Geometry check sheet. Reference: the model listing, model coordinates, mm. Give positions to 0.01 mm unless a question says otherwise; leave off trailing zeros. Order: outer loops, then holes, each group sorted by start corner. A loop starts at its lowest first (then second) coordinate and runs counter-clockwise, first axis right, second up.
Autodesk Inventor part; units mm, degrees
ref_plane "YZ Plane" through (0, 0, 0) normal (1, 0, 0) x (0, 1, 0)
ref_plane "XZ Plane" through (0, 0, 0) normal (0, 1, 0) x (-1, 0, 0)
ref_plane "XY Plane" through (0, 0, 0) normal (0, 0, 1) x (1, 0, 0)
sketch "Sketch1" plane through (0, 0, 0) normal (0, 0, 1) x (1, 0, 0)
  line L0 (0, 0) -> (0, 6.35)
  line L1 (0, 6.35) -> (97.04, 6.35)
  line L2 (97.04, 6.35) -> (97.04, 0)
  line L3 (97.04, 0) -> (0, 0)
  dimension "d0" = 6.35
  dimension "d1" = 97.04
extrude "Extrusion1" add sketch "Sketch1" along normal blind 332
sketch "Sketch2" plane through (0, 0, 332) normal (0, 0, 1) x (1, 0, 0)
  line L0 (0, 0) -> (16.1733, 0) construction
  line L1 (16.1733, 0) -> (48.52, 0) construction
  line L2 (48.52, 0) -> (80.8667, 0) construction
  line L3 (0, 0) -> (97.04, 0)
  arc A0 (19.3483, 0) -> (12.9983, 0) centre (16.1733, 0) ccw
  arc A1 (51.695, 0) -> (45.345, 0) centre (48.52, 0) ccw
  arc A2 (84.0417, 0) -> (77.6917, 0) centre (80.8667, 0) ccw
  line L4 (12.9983, 0) -> (19.3483, 0)
  line L5 (45.345, 0) -> (51.695, 0)
  line L6 (77.6917, 0) -> (84.0417, 0)
  dimension "d4" = 16.1733
  dimension "d5" = 32.3467
  dimension "d6" = 32.3467
  dimension "d12" = 3.175
  dimension "d13" = 3.175
  dimension "d14" = 3.175
extrude "Extrusion3" cut sketch "Sketch2" against normal through all
sketch "Sketch3" plane through (0, 0, 332) normal (0, 0, 1) x (1, 0, 0)
  arc A0 (19.3483, 0) -> (12.9983, 0) centre (16.1733, 0) ccw
  line L0 (0, 0) -> (0, 6.35) construction
  line L1 (0, 0) -> (0, 3.175) construction
  arc A1 (19.3483, 0) -> (12.9983, 0) centre (16.1733, 0) ccw construction
  line L2 (16.1733, 3.175) -> (12.9983, 3.175)
  line L3 (0, 3.175) -> (6.4992, 3.175) construction
  line L4 (45.345, 0) -> (19.3483, 0) construction
  line L5 (19.3483, 0) -> (32.3467, 0) construction
  circle A2 centre (32.3467, 3.175) radius 1.5
  circle A3 centre (6.4992, 3.175) radius 1.5
  line L6 (51.695, 0) -> (64.6933, 0) construction
  line L7 (77.6917, 0) -> (51.695, 0) construction
  circle A4 centre (64.6933, 3.175) radius 1.5
  line L8 (84.0417, 0) -> (90.5408, 0) construction
  line L9 (97.04, 0) -> (84.0417, 0) construction
  circle A5 centre (90.5408, 3.175) radius 1.5
  dimension "d17" = 3
  dimension "d18" = 3
  dimension "d19" = 3
  dimension "d20" = 3
extrude "Extrusion4" cut sketch "Sketch3" against normal blind 20
sketch "Sketch4" plane through (0, 0, 0) normal (0, 0, -1) x (-1, 0, 0)
  circle A0 centre (-6.4992, 3.175) radius 1.5
  circle A1 centre (-32.3467, 3.175) radius 1.5
  circle A2 centre (-64.6933, 3.175) radius 1.5
  circle A3 centre (-90.5408, 3.175) radius 1.5
  dimension "d23" = 3
  dimension "d24" = 3
  dimension "d25" = 3
  dimension "d26" = 3
extrude "Extrusion5" cut sketch "Sketch4" against normal blind 20
sketch "Sketch5" plane through (0, 0, 332) normal (0, 0, 1) x (1, 0, 0)
  circle A0 centre (64.6933, 3.175) radius 1.5
  circle A1 centre (32.3467, 3.175) radius 1.5
  circle A2 centre (6.4992, 3.175) radius 1.5
  circle A3 centre (90.5408, 3.175) radius 1.5
  arc A4 (51.695, 0) -> (45.345, 0) centre (48.52, 0) ccw
  line L0 (51.695, 0) -> (77.6917, 0)
  arc A5 (84.0417, 0) -> (77.6917, 0) centre (80.8667, 0) ccw
  line L1 (84.0417, 0) -> (97.04, 0)
  line L2 (97.04, 0) -> (97.04, 6.35)
  line L3 (97.04, 6.35) -> (0, 6.35)
  line L4 (0, 6.35) -> (0, 0)
  line L5 (0, 0) -> (12.9983, 0)
  arc A6 (19.3483, 0) -> (12.9983, 0) centre (16.1733, 0) ccw
  line L6 (19.3483, 0) -> (45.345, 0)
extrude "Extrusion6" add sketch "Sketch5" along normal blind 30.87
sketch "Sketch6" plane through (0, 0, 362.87) normal (0, 0, 1) x (1, 0, 0)
  circle A0 centre (90.5408, 3.175) radius 1.5
  circle A1 centre (6.4992, 3.175) radius 1.5
  circle A2 centre (32.3467, 3.175) radius 1.5
  circle A3 centre (64.6933, 3.175) radius 1.5
  arc A4 (51.695, 0) -> (45.345, 0) centre (48.52, 0) ccw
  line L0 (51.695, 0) -> (77.6917, 0)
  arc A5 (84.0417, 0) -> (77.6917, 0) centre (80.8667, 0) ccw
  line L1 (84.0417, 0) -> (97.04, 0)
  line L2 (97.04, 0) -> (97.04, 6.35)
  line L3 (97.04, 6.35) -> (0, 6.35)
  line L4 (0, 6.35) -> (0, 0)
  line L5 (0, 0) -> (12.9983, 0)
  arc A6 (19.3483, 0) -> (12.9983, 0) centre (16.1733, 0) ccw
  line L6 (19.3483, 0) -> (45.345, 0)
extrude "Extrusion7" cut sketch "Sketch6" against normal blind 6.35
properties part number "coverplate"
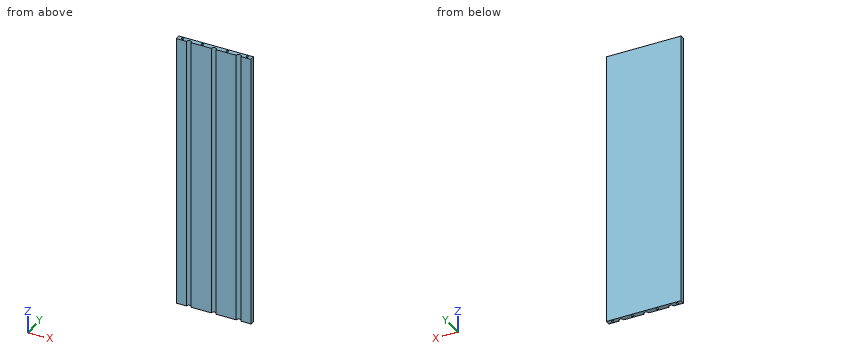
Item 1: Sectioned sample at B-B (x = 48.52). Enter the section's corners in (y, z) (3 decimals), and give its area (3 significant figures).
Reported:
outline: (3.175, 0) - (6.35, 0) - (6.35, 356.52) - (3.175, 356.52) - close
area: 1,130 mm2
Item 2: Gauge pin test, flat ends, axial feed: pin 1 (2.5 mm diameter, centred on x = 32.35, y = 3.18, fed in from +Z); pin 2 (0.9 mm diameter, centred on x = 65, y = 3.5, fed in from -Z). Record the tip position at first contact, or that the pin passes through.
Reported:
pin 1: stops at z = 312
pin 2: stops at z = 20
Item 3: Scan lines: L1, parallel to X at y = 1.5, z = 227; L2, parallel to X at y = 1.75, z = 214.5; L3, parallel to Y at x = 48, z = 64.5. Record each from-to range of solid material in increasing order.
Reported:
L1: x = 0 to 13.37, 18.97 to 45.72, 51.32 to 78.07, 83.67 to 97.04
L2: x = 0 to 13.52, 18.82 to 45.87, 51.17 to 78.22, 83.52 to 97.04
L3: y = 3.13 to 6.35
Item 4: Sectioned sample at A-A (z = 261.5). Enter the section's corners in (x, y) (3 decimals), and give its area (3 significant figures).
Reported:
outline: (0, 0) - (12.998, 0) arc R3.175 cw to (19.348, 0) - (45.345, 0) arc R3.175 cw to (51.695, 0) - (77.692, 0) arc R3.175 cw to (84.042, 0) - (97.04, 0) - (97.04, 6.35) - (0, 6.35) - close
area: 569 mm2
